Input: part model. Units: mm. Frame: model coordinates. Face numbers are marked on the shaded views. A direction names the side the tool comes from. Give positions to 0.01 mm unless a question says otherwise; leave off trailing zeros. Write each loop counter-clockwise with the first axis right and the second up, starting at its lowest first coordinate (ties: lowest second). Pieces come first, ordered by that corner, then holes. Notation, with made-up numbers: (-6.5, 55) - (10.5, 55) arc R11 ccw to (10.5, 67) - close; hole circle Ø4 at (46, 16). An arc over 180 degrees is marked (long way). Use a Markdown table: item, result. Add a question column.
1. Pin query (flat end, axial travel): pin 1 (5 mm diameter, centred on y = 44.5, z = 19, fed in from +X); pin 2 (6 mm diameter, centred on x = -35, z = 26, fed in from -Y); pin 3 (1.5 mm diameter, centred on x = 63, z = 22.5, fed in from -Y). Return the tip coordinate at first contact, or that it passes through.
2. Section query A-A, the plane z = 25.5. Return loops of the section in (x, y).
3. Section query B-B, the plane y = -77. Return loops of the section in (x, z), plus the area to 3 significant figures.
4. Material intervals for probe 1 along Z at (x, y) = (12, -2.5); probe 2 along Y at (x, z) = (-48.5, 17); probe 3 along Y at (x, z) = (-39, 1.5), sorted ascending.
5. Set-up query: the marked faces 1 and 2. Return all of +Z, -Z, +X, -X, +Y, -Y with unobstructed straight access to the full face (end or side cutting, diameter ignored); none if empty.
```python
from build123d import *

# Parameters (mm, degrees)
BASE_FLANGE1_DEPTH            = 4
EDGE_FLANGE1_STRIP_W          = 16.4
EDGE_FLANGE1_STRIP_H          = 4
EDGE_FLANGE1_STRIP_CUT_DEPTH  = 240.587208925
EDGE_FLANGE1_RELIEF_W         = 18.4
EDGE_FLANGE1_RELIEF_H         = 2
EDGE_FLANGE1_RELIEF_CUT_DEPTH = 4
EDGE_FLANGE1_DEPTH            = 240.587208925
SKETCH9_R                     = 3
CUT_EXTRUDE1_DEPTH            = 10


# Sheet-metal steps are written as plain solids
with BuildPart() as part:
    # Sketch1 → Base-Flange1 (new body)
    with BuildSketch(Plane.XY):
        Polygon((88.217940857, -94.952805993), (-98.507333634, 101.415804733), (-97.402972414, 107.112654424), (-68.257223266, 120.395137548), (97.52878242, -53.952805993), (97.52878242, -89.952805993), (92.52878242, -94.952805993), align=None)
    extrude(amount=-BASE_FLANGE1_DEPTH)

    # Edge-Flange1 strip (across the edge) → Edge-Flange1 strip cut (cut)
    with BuildSketch(Plane(origin=(97.52878242, -53.952805993, 0), x_dir=(-0.7246766954889595, -0.689089026915392, 3.4914813388431334e-15), z_dir=(-0.689089026915392, 0.7246766954889595, 0))):
        with Locations((-4, -2)):
            Rectangle(EDGE_FLANGE1_STRIP_W, EDGE_FLANGE1_STRIP_H)
    extrude(amount=EDGE_FLANGE1_STRIP_CUT_DEPTH, mode=Mode.SUBTRACT)

    # Edge-Flange1 relief (on the sheet) → Edge-Flange1 relief cut (cut)
    with BuildSketch(Plane(origin=(94.485140299, -56.846979906, 0), x_dir=(-0.7246766954889595, -0.689089026915392, 6.982962677686267e-15), z_dir=(0, 0, 1))):
        with Locations((-7.2, 1)):
            Rectangle(EDGE_FLANGE1_RELIEF_W, EDGE_FLANGE1_RELIEF_H)
        with Locations((-7.2, -241.587208925)):
            Rectangle(EDGE_FLANGE1_RELIEF_W, EDGE_FLANGE1_RELIEF_H)
    extrude(amount=-EDGE_FLANGE1_RELIEF_CUT_DEPTH, mode=Mode.SUBTRACT)

    # Edge-Flange1 section (across the edge) → Edge-Flange1 (add)
    with BuildSketch(Plane(origin=(97.52878242, -53.952805993, 0), x_dir=(-0.7246766954889595, -0.689089026915392, 3.4914813388431334e-15), z_dir=(-0.689089026915392, 0.7246766954889595, 0))):
        with BuildLine():
            Line((0, 0.2), (0, 31))
            Line((0, 31), (4, 31))
            Line((4, 31), (4, 0.2))
            ThreePointArc((4, 0.2), (4.058578644, 0.058578644), (4.2, 0))
            Line((4.2, 0), (4.2, -4))
            ThreePointArc((4.2, -4), (1.230151519, -2.769848481), (0, 0.2))
        make_face()
    extrude(amount=EDGE_FLANGE1_DEPTH)

    # Sketch9 → Cut-Extrude1 (cut)
    with BuildSketch(Plane(origin=(24.275617922, 23.083482656, 0), x_dir=(0, 0, -1), z_dir=(0.7246766954889596, 0.689089026915392, -3.4889229979583694e-15))):
        with Locations(Location((-13.5, 99.282853991, 0), (0, 0, 90))):
            Circle(SKETCH9_R)
    extrude(amount=-CUT_EXTRUDE1_DEPTH, mode=Mode.SUBTRACT)


solid = part.part
```
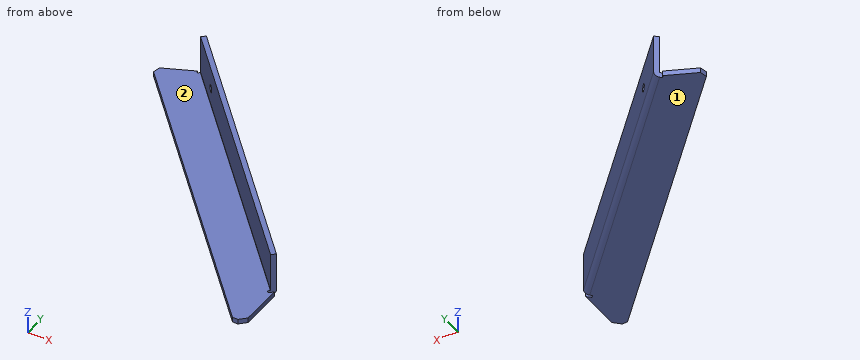
Result sheet:
| question | item | result |
|---|---|---|
| 1 | pin 1 | stops at x = 6.29 |
| 1 | pin 2 | stops at y = 76.46 |
| 1 | pin 3 | stops at y = -24.23 |
| 2 | outline | (-71.16, 117.64) - (94.63, -56.71) - (97.53, -53.95) - (-68.26, 120.4) - close |
| 3 | outline | (71.15, -4) - (97.53, -4) - (97.53, 0) - (71.15, 0) - close |
| 3 | area | 106 mm² |
| 4 | probe 1 | z = -4 to 0 |
| 4 | probe 2 | y = 93.81 to 99.62 |
| 4 | probe 3 | y = 83.82 to 89.63 |
| 5 | face 1 | -Z, +X, -X, +Y, -Y |
| 5 | face 2 | +Z, -X, -Y |
